```python
from build123d import *

# Parameters (mm, degrees)
SKETCH1_W            = 111.9
SKETCH1_H            = 42
BOSS_EXTRUDE1_DEPTH  = 5
SKETCH2_W            = 6.5
SKETCH2_H            = 6.5
BOSS_EXTRUDE2_DEPTH  = 3.5
CUT_EXTRUDE1_DEPTH   = 2
CUT_EXTRUDE2_DEPTH   = 2
BOSS_EXTRUDE3_DEPTH  = 3.5
FILLET1_R            = 0.2
FILLET1_OF_MIRROR1_R = 0.2
FILLET2_R            = 1.5
FILLET3_R            = 0.5
FILLET4_R            = 0.2
FILLET5_R            = 0.2
FILLET6_R            = 0.2


with BuildPart() as part:
    # Sketch1 → Boss-Extrude1 (new body)
    with BuildSketch(Plane.XY):
        Rectangle(SKETCH1_W, SKETCH1_H)
    extrude(amount=BOSS_EXTRUDE1_DEPTH)

    # Sketch2 → Boss-Extrude2 (add)
    with BuildSketch(Plane(origin=(0, 0, 0), x_dir=(-1, 0, 0), z_dir=(0, 0, -1))):
        with Locations((52.7, 17.75)):
            Rectangle(SKETCH2_W, SKETCH2_H)
        with Locations((-52.7, -17.75)):
            Rectangle(SKETCH2_W, SKETCH2_H)
    extrude(amount=BOSS_EXTRUDE2_DEPTH)

    # Sketch3 → Cut-Extrude1 (cut)
    with BuildSketch(Plane(origin=(0, 0, 0), x_dir=(-1, 0, 0), z_dir=(0, 0, -1))):
        Polygon((-45.45, -17), (51.95, -17), (51.95, 10.5), (45.45, 10.5), (45.45, 17), (-51.95, 17), (-51.95, -10.5), (-45.45, -10.5), align=None)
        Polygon((-42.45, -14), (48.95, -14), (48.95, 7.5), (42.45, 7.5), (42.45, 14), (-48.95, 14), (-48.95, -7.5), (-42.45, -7.5), align=None, mode=Mode.SUBTRACT)
    extrude(amount=-CUT_EXTRUDE1_DEPTH, mode=Mode.SUBTRACT)

    # Sketch5 → Cut-Extrude2 (cut)
    with BuildSketch(Plane(origin=(0, 0, 0), x_dir=(-1, 0, 0), z_dir=(0, 0, -1))):
        Polygon((-40.45, -12), (46.95, -12), (46.95, 5.5), (40.45, 5.5), (40.45, 12), (-46.95, 12), (-46.95, -5.5), (-40.45, -5.5), align=None)
    extrude(amount=-CUT_EXTRUDE2_DEPTH, mode=Mode.SUBTRACT)

    # Sketch6 → Boss-Extrude3 (add, symmetric)
    with BuildSketch(Plane(origin=(0, 0, 0), x_dir=(-1, 0, 0), z_dir=(0, -1, 0))):
        Polygon((53.95, 5), (51.95, 7), (48.95, 7), (48.95, 0), (48.95, -2), (51.95, -2), (51.95, 0), (51.95, 3), align=None)
    boss_extrude3 = extrude(amount=BOSS_EXTRUDE3_DEPTH, both=True)

    # Fillet1
    fillet1_edges = [part.edges().sort_by_distance(p)[0] for p in [
        (-51.95, 3.5, -1.5),
        (-48.95, 0, -7),
        (-52.95, 3.5, -6),
        (-53.95, 0, -5),
        (-50.45, 3.5, -7),
        (-51.95, 0, -7),
        (-52.95, 3.5, -4),
        (-51.95, 0, -3),
        (-48.95, 3.5, -3.5),
    ]]
    fillet(fillet1_edges, radius=FILLET1_R)

    # Mirror1: Boss-Extrude3 across plane
    add(boss_extrude3.mirror(Plane.ZY))

    # Fillet1 of Mirror1
    fillet1_of_mirror1_edges = [part.edges().sort_by_distance(p)[0] for p in [
        (51.95, 3.5, -1.5),
        (48.95, 0, -7),
        (52.95, 3.5, -6),
        (53.95, 0, -5),
        (50.45, 3.5, -7),
        (51.95, 0, -7),
        (52.95, 3.5, -4),
        (51.95, 0, -3),
        (48.95, 3.5, -3.5),
    ]]
    fillet(fillet1_of_mirror1_edges, radius=FILLET1_OF_MIRROR1_R)

    # Fillet2
    fillet2_edges = [part.edges().sort_by_distance(p)[0] for p in [
        (-55.95, 21, 0.75),
        (55.95, 21, 2.5),
        (55.95, -21, 0.75),
        (-55.95, -21, 2.5),
    ]]
    fillet(fillet2_edges, radius=FILLET2_R)

    # Fillet3
    fillet3_edges = [part.edges().sort_by_distance(p)[0] for p in [
        (0, -21, 5),
        (-55.95, 0, 5),
        (55.95, 0, 5),
        (0, 21, 5),
        (55.510660172, 20.560660172, 5),
        (55.510660172, -20.560660172, 5),
        (-55.510660172, 20.560660172, 5),
        (-55.510660172, -20.560660172, 5),
    ]]
    fillet(fillet3_edges, radius=FILLET3_R)

    # Fillet4
    fillet4_edges = [part.edges().sort_by_distance(p)[0] for p in [
        (43.7, -5.5, 2),
        (46.95, 3.25, 2),
        (3.25, 12, 2),
        (-40.45, 8.75, 2),
        (-43.7, 5.5, 2),
        (-46.95, -3.25, 2),
        (-3.25, -12, 2),
        (40.45, -8.75, 2),
        (3.25, 17, 2),
        (-45.45, 13.75, 2),
        (-48.7, 10.5, 2),
        (-51.95, 7, 2),
        (-50.45, 3.5, 2),
        (-48.95, 5.5, 2),
        (-45.7, 7.5, 2),
        (-42.45, 10.75, 2),
        (3.25, 14, 2),
        (48.95, 8.75, 2),
        (50.45, 3.5, 2),
        (51.95, 10.25, 2),
        (48.95, -5.5, 2),
        (45.7, -7.5, 2),
        (42.45, -10.75, 2),
        (-3.25, -14, 2),
        (-48.95, -8.75, 2),
        (-50.45, -3.5, 2),
        (-51.95, -10.25, 2),
        (-3.25, -17, 2),
        (45.45, -13.75, 2),
        (48.7, -10.5, 2),
        (51.95, -7, 2),
        (50.45, -3.5, 2),
        (51.95, -3.5, 1),
        (48.95, -3.5, 1),
        (51.95, 3.5, 1),
        (48.95, 3.5, 1),
        (-48.95, -3.5, 1),
        (-51.95, -3.5, 1),
        (-48.95, 3.5, 1),
        (-51.95, 3.5, 1),
        (-51.95, -17, 1),
    ]]
    fillet(fillet4_edges, radius=FILLET4_R)

    # Fillet5
    fillet5_edges = [part.edges().sort_by_distance(p)[0] for p in [
        (51.95, -3.5, -1.458578644),
        (51.965224093, -3.5, -2.993693974),
        (52.908578644, -3.5, -3.958578644),
        (53.867157288, -3.5, -5),
        (52.908578644, -3.5, -6.041421356),
        (51.943693974, -3.5, -6.984775907),
        (50.508578644, -3.5, -7),
        (49.008578644, -3.5, -6.941421356),
        (-51.95, -3.5, -1.458578644),
        (-51.965224093, -3.5, -2.993693974),
        (-52.908578644, -3.5, -3.958578644),
        (-53.867157288, -3.5, -5),
        (-52.908578644, -3.5, -6.041421356),
        (-51.943693974, -3.5, -6.984775907),
        (-50.508578644, -3.5, -7),
        (-49.008578644, -3.5, -6.941421356),
        (48.95, -3.5, -3.4),
        (-48.95, -3.5, -3.4),
    ]]
    fillet(fillet5_edges, radius=FILLET5_R)

    # Fillet6
    fillet6_edges = [part.edges().sort_by_distance(p)[0] for p in [
        (-55.95, 17, -3.5),
        (55.95, -17, -3.5),
        (51.95, -21, -3.5),
        (-51.95, 21, -3.5),
        (-55.510660172, 20.560660172, -3.5),
        (55.510660172, -20.560660172, -3.5),
    ]]
    fillet(fillet6_edges, radius=FILLET6_R)


solid = part.part
```
Geometry check sheet. Reference: the model listing, model coordinates, mm. A direction names the side the tool comes from. Round coordinates to 2 decimals unless told otherwise and drop trailing zeros. Write each loop counter-clockwise with the first axis right and the second up, starting at its lowest first coordinate (ties: lowest second). Pieces come first, ordered by that corner, then holes. Notation, with made-up numbers: (8, 4.25) - (43, 4.25) arc R17 cw to (43, 26.25) - close; hole circle Ø6 at (34.25, 28.5). An arc over 180 degrees is marked (long way). Write each question's results on one line, items separated by ' | '.
(1) Depth check by flat-ended pin: pin 1 Ø1.4 at (x, z) = (52, -4.5) entering from +Y; pin 2 Ø4 at (x, y) = (-5, 1) entering from -Z; pin 3 Ø3 at (y, z) = (-18, -2.5) entering from -X. Enter the tip coordinate at first touch or a pass-through.
Computed:
pin 1: stops at y = 3.5 | pin 2: stops at z = 2 | pin 3: stops at x = 49.45
(2) Sectioned sample at D-D, the plane y = -9. Enter the section's corners in (x, z), plus the area to 3 significant figures.
Computed:
outline: (-55.95, 0) - (-51.95, 0) - (-51.95, 1.8) arc R0.2 cw to (-51.75, 2) - (-49.15, 2) arc R0.2 cw to (-48.95, 1.8) - (-48.95, 0) - (-46.95, 0) - (-46.95, 1.8) arc R0.2 cw to (-46.75, 2) - (40.25, 2) arc R0.2 cw to (40.45, 1.8) - (40.45, 0) - (42.45, 0) - (42.45, 1.8) arc R0.2 cw to (42.65, 2) - (51.75, 2) arc R0.2 cw to (51.95, 1.8) - (51.95, 0) - (55.95, 0) - (55.95, 4.5) arc R0.5 ccw to (55.45, 5) - (-55.45, 5) arc R0.5 ccw to (-55.95, 4.5) - close | area: 360 mm^2
(3) Sectioned sample at C-C, the plane x = 4.5. Enter the section's corners in (y, z), plus the area to 3 significant figures.
Computed:
outline: (-21, 0) - (-17, 0) - (-17, 1.8) arc R0.2 cw to (-16.8, 2) - (-14.2, 2) arc R0.2 cw to (-14, 1.8) - (-14, 0) - (-12, 0) - (-12, 1.8) arc R0.2 cw to (-11.8, 2) - (11.8, 2) arc R0.2 cw to (12, 1.8) - (12, 0) - (14, 0) - (14, 1.8) arc R0.2 cw to (14.2, 2) - (16.8, 2) arc R0.2 cw to (17, 1.8) - (17, 0) - (21, 0) - (21, 4.5) arc R0.5 ccw to (20.5, 5) - (-20.5, 5) arc R0.5 ccw to (-21, 4.5) - close | area: 150 mm^2
(4) Sectioned sample at B-B, the plane y = 13. Enter the section's corners in (x, z).
Computed:
outline: (-55.95, 0) - (-45.45, 0) - (-45.45, 1.8) arc R0.2 cw to (-45.25, 2) - (-42.65, 2) arc R0.2 cw to (-42.45, 1.8) - (-42.45, 0) - (48.95, 0) - (48.95, 1.8) arc R0.2 cw to (49.15, 2) - (51.75, 2) arc R0.2 cw to (51.95, 1.8) - (51.95, 0) - (55.95, 0) - (55.95, 4.5) arc R0.5 ccw to (55.45, 5) - (-55.45, 5) arc R0.5 ccw to (-55.95, 4.5) - close
(5) Set-up check for faces 1 (the face through (52.88, 3.44, -4.01)), 2 (the face through (-53, 14.5, -2)), 3 (the face through (-52.88, -3.44, -4.01)), 4 (the face through (49.45, -18, -2)): record each of +Z, -Z, +X, -X, +Y, -Y from which the full face is reachable in a straight line by a thin tool's end or side.
Computed:
face 1: +X, +Y | face 2: -Z, +X, -X | face 3: -X, -Y | face 4: -Z, -X, -Y
(6) Draft check along X on faces 5 (the face through (-48.95, 0, -3)), 6 (the face through (51.95, 0, -1)), 7 (the face through (-51.95, 0, -1)). Enter one of: pulls with the +X half, pulls with the -X half, needs draft (parallel to the pull), parting line crosses it, or undercut.
Computed:
face 5: undercut | face 6: pulls with the +X half | face 7: pulls with the -X half
(7) Thickness scan on probe 1 along Y at (x, z) = (0.5, 1.75); probe 2 along Y at (x, z) = (-49.5, 1.75); probe 3 along X at (y, z) = (6, 1.5). Record the ranges inside material, lowest first. Write a range as from..to.
Computed:
probe 1: y = -21..-17, -14..-12, 12..14, 17..21 | probe 2: y = -21..-17, -3.5..3.5, 10.5..21 | probe 3: x = -55.95..-51.95, -48.95..-40.45, 46.95..48.95, 51.95..55.95
(8) Sectioned sample at A-A, the plane z = -1. Enter the section's corners in (x, y).
Computed:
outline: (-55.95, 14.5) - (-49.45, 14.5) - (-49.45, 21) - (-54.45, 21) arc R1.5 ccw to (-55.95, 19.5) - close; (-51.95, -3.3) arc R0.2 ccw to (-51.75, -3.5) - (-49.15, -3.5) arc R0.2 ccw to (-48.95, -3.3) - (-48.95, 3.3) arc R0.2 ccw to (-49.15, 3.5) - (-51.75, 3.5) arc R0.2 ccw to (-51.95, 3.3) - close; (48.95, -3.3) arc R0.2 ccw to (49.15, -3.5) - (51.75, -3.5) arc R0.2 ccw to (51.95, -3.3) - (51.95, 3.3) arc R0.2 ccw to (51.75, 3.5) - (49.15, 3.5) arc R0.2 ccw to (48.95, 3.3) - close; (49.45, -21) - (54.45, -21) arc R1.5 ccw to (55.95, -19.5) - (55.95, -14.5) - (49.45, -14.5) - close
